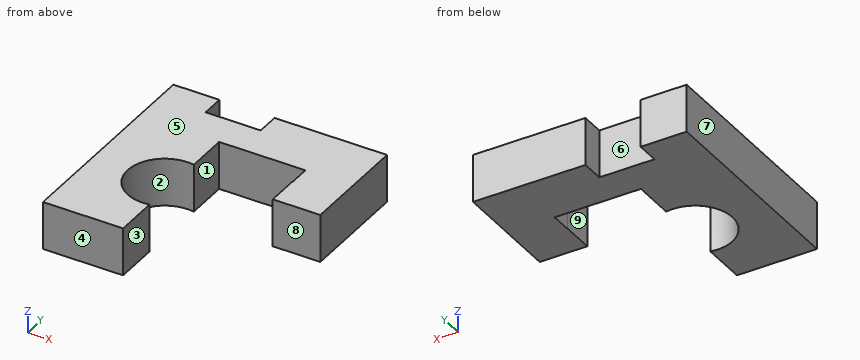
from build123d import *

# Parameters (mm, degrees)
F1_DEPTH = 2


with BuildPart() as f1:
    # F0 (on Top) → F1 (new body)
    with BuildSketch(Plane.XY):
        with BuildLine():
            Line((0, 9), (0, 0))
            Line((0, 0), (3.343781, 0))
            Line((3.343781, 0), (3.343781, 1.832761))
            ThreePointArc((3.343781, 1.832761), (1.502494, 3.357977), (3.343781, 4.883193))
            Line((3.343781, 4.883193), (3.343781, 6.628936))
            Line((3.343781, 6.628936), (6.945667, 6.628936))
            Line((6.945667, 6.628936), (6.945667, 5.751214))
            Line((6.945667, 5.751214), (6.931864, 5.751214))
            Line((6.931864, 5.751214), (6.931864, 4.395805))
            Line((6.931864, 4.395805), (8.91781, 4.395805))
            Line((8.91781, 4.395805), (8.91781, 9))
            Line((8.91781, 9), (4.224609, 9))
            Line((4.224609, 9), (4.224609, 8.044908))
            Line((4.224609, 8.044908), (1.923485, 8.044908))
            Line((1.923485, 8.044908), (1.923485, 9))
            Line((1.923485, 9), (0, 9))
        make_face()
    extrude(amount=F1_DEPTH)


solid = f1.part
Geometry: final body of the model. Coordinates: model frame, mm. Face numbers are marked on the shaded views. A direction names the side the tool comes from. Give positions to 0.01 mm unless a question says otherwise; leave off trailing zeros. Loops run counter-clockwise (first coordinate to the right, second up) from the corner with the lowest first, then second, coordinate; pieces in that order, holes last. Notation, with made-up numbers: (54.25, 26) - (62.25, 26) arc R35 ccw to (62.25, 59) - close; hole circle Ø6 at (83, -3.5). An arc over 180 degrees is marked (long way). Answer as CSV lines item,"result". Start each with the question number.
1. Section D-D, the plane x = 5. Return loops of the section in (y, z).
2. Section A-A, the plane y = 8.25. Return loops of the section in (x, z).
3. Draft query along X for the marked faces 1, 2, 3 and 4. Return one class per face: released by +X, released by -X, zero draft, split by the parting line, or undercut.
4. Reachability of the marked faces 5, 6, 7, 8 and 9 from +Z, -Z, +X, -X, +Y, -Y: full face, straight path, thin tool, end or side. Return the list, or none.
5. Ray query, L1, parallel to X at y = 5.5, z = 1.05; L2, parallel to Y at x = 3, z = 0.9; L3, parallel to Y at x = 8.75, z = 0.1. Return the intervals inside material, ascending.
6. Pin query (flat end, axial travel): P1, Ø1, axis at x = 6, z = 1, coming from the -Y side; P2, Ø1, axis at x = 3.5, z = 1.5, coming from the +Y side. Return the tip coordinate at first contact, or that it passes through.
7. Section B-B, the plane x = 2.5. Return loops of the section in (y, z), plus the area to 3 significant figures.
Answers:
1,outline,"(6.63, 0) - (9, 0) - (9, 2) - (6.63, 2) - close"
2,outline,"(0, 0) - (1.92, 0) - (1.92, 2) - (0, 2) - close; (4.22, 0) - (8.92, 0) - (8.92, 2) - (4.22, 2) - close"
3,face 1,"undercut"
3,face 2,"undercut"
3,face 3,"released by +X"
3,face 4,"zero draft"
4,face 5,"+Z, +X, -X, +Y, -Y"
4,face 6,"+Z, -Z, +Y"
4,face 7,"+Z, -Z, -X, +Y, -Y"
4,face 8,"+Z, -Z, +X, -Y"
4,face 9,"+Z, -Z, -Y"
5,L1,"x = 0 to 3.34, 6.93 to 8.92"
5,L2,"y = 0 to 1.81, 4.91 to 8.04"
5,L3,"y = 4.4 to 9"
6,P1,"stops at y = 6.63"
6,P2,"stops at y = 8.04"
7,outline,"(0, 0) - (1.91, 0) - (1.91, 2) - (0, 2) - close; (4.81, 0) - (8.04, 0) - (8.04, 2) - (4.81, 2) - close"
7,area,"10.3 mm2"
